Solid Edge part; units mm, degrees
sketch "Sketch1" plane through (0, 0, 0) normal (0, -1, 0) x (1, 0, 0)
  line L0 (-11, -3.5) -> (-13.6449, 11.5)
  line L1 (-13.6449, 11.5) -> (-21.7683, 11.5)
  line L2 (-21.7683, 11.5) -> (-17.7128, -11.5)
  line L3 (-17.7128, -11.5) -> (17.7128, -11.5)
  line L4 (17.7128, -11.5) -> (21.7683, 11.5)
  line L5 (21.7683, 11.5) -> (13.6449, 11.5)
  line L6 (13.6449, 11.5) -> (11, -3.5)
  line L7 (11, -3.5) -> (-11, -3.5)
extrude "Protrusion1" add sketch "Sketch1" against normal blind 20
sketch "Sketch2" plane through (0, 0, 0) normal (0, -1, 0) x (1, 0, 0)
  arc A0 (-9, -11.5) -> (9, -11.5) centre (0, -11.5) ccw
  line L0 (-9, -11.5) -> (9, -11.5)
extrude "ExtrudedCutout_1" add sketch "Sketch2" against normal blind 20
hole "Trou_pivot" at (0, 0, -11.5) direction (0, 1, 0) diameter 9 end up to next
fillet "Congé_2mm" radius 2 8 edges at (0, 0, -3.5) (-12.3225, 0, 4) (-12.3225, 20, 4) (12.3225, 0, 4) (0, 20, -3.5) (12.3225, 20, 4) (-13.6449, 10, 11.5) (13.6449, 10, 11.5)
properties material "Polyuréthane"
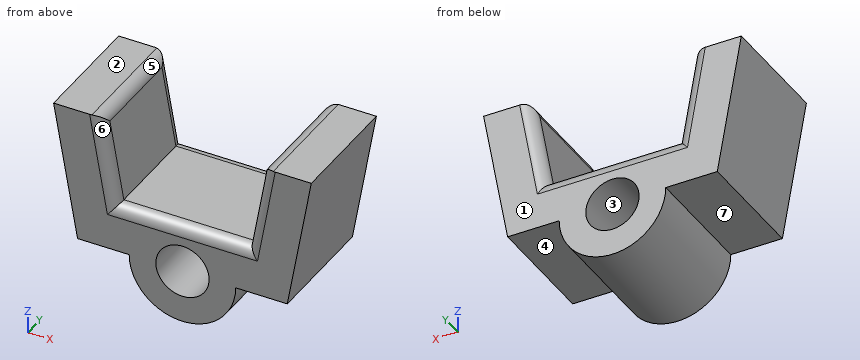
Read the model definition and answer for the solid it produces. Units are mm, in the model's axes. Face numbers are marked on the shaded views. A direction names the side the tool comes from. Round coordinates to 2 decimals unless told otherwise and drop trailing zeros. Loops run counter-clockwise (first coordinate to the right, second up) from the corner with the lowest first, then second, coordinate; pieces in that order, holes last. Notation, with made-up numbers: (80, 82) - (115, 82) arc R32 cw to (115, 121) - close; hole circle Ø4 at (82, 2.25). An arc over 180 degrees is marked (long way). One line per question, with ' | ' between items. Start each with the question number.
Q1. Section B-B on y = 17 is taken. Give the vertices of the cut face in (x, z), plus the area to 3 significant figures.
Q2. Flat-ended cylindrical pins translate along their axes: pin 1 (4.5 mm diameter, centred on x = -13, y = 6, fed in from -Z); pin 2 (12 mm diameter, centred on x = -13.5, y = 9.5, fed in from -Z); pin 3 (6 mm diameter, centred on y = 7, z = -15.5, fed in from +X). Find the tip coordinate at first contact, or state that the pin passes through.
Q3. For the marked faces 4, 5, 6 and 7, determine the directions among +Z, -Z, +X, -X, +Y, -Y from which every point of the face is accessible in a straight line to the end or side of a thin tool.
Q4. Section C-C on z = -9 is taken. Give the vertices of the cut face in (x, y).
Q5. For a pull along Z with two mould halves and no side action, classify the marked faces 1, 2 and 3 as +Z half, -Z half, draft (parallel to the pull), parting line (faces both ways), or undercut.
Q6. Section A-A on x = 0 is taken. Give the vertices of the cut face in (y, z).
Q7. Section D-D on x = 10.5 is taken. Give the vertices of the cut face in (y, z), plus the area to 3 significant figures.
Q8. Find the intervals of material crossed by L1, parallel to Z at x = 0, y = 16.25; L2, parallel to Z at x = 17, y = 7.25; L3, parallel to X at y = 17, z = -9.5, in increasing order.
Established:
1) outline: (-21.77, 11.5) - (-17.71, -11.5) - (-9, -11.5) arc R9 ccw to (9, -11.5) - (17.71, -11.5) - (21.77, 11.5) - (15.32, 11.5) arc R2 ccw to (13.35, 9.85) - (11, -3.5) - (-11, -3.5) - (-13.35, 9.85) arc R2 ccw to (-15.32, 11.5) - close; hole circle Ø9 at (0, -11.5) | area: 601 mm²
2) pin 1: z = -11.5 | pin 2: z = -16.47 | pin 3: x = 8.94
3) face 4: -Z, +X, +Y, -Y | face 5: +Z, +Y, -Y | face 6: +Z, -Y | face 7: -Z, -X, +Y, -Y
4) outline: (-18.15, 0) - (-3.74, 0) - (-3.74, 20) - (-18.15, 20) - close; (3.74, 0) - (18.15, 0) - (18.15, 20) - (3.74, 20) - close
5) face 1: draft | face 2: +Z half | face 3: undercut
6) outline: (0, -20.5) - (20, -20.5) - (20, -16) - (0, -16) - close; (0, -7) - (20, -7) - (20, -5.5) arc R2 ccw to (18, -3.5) - (2, -3.5) arc R2 ccw to (0, -5.5) - close
7) outline: (0, -11.5) - (20, -11.5) - (20, -5.5) arc R2 ccw to (18, -3.5) - (2, -3.5) arc R2 ccw to (0, -5.5) - close | area: 158 mm²
8) L1: -20.5 to -16, -7 to -3.5 | L2: -11.5 to 11.5 | L3: -18.07 to -4.03, 4.03 to 18.07
